Check sheet for the drawn part. Datum: minimum x, y, z corner. Units: mm. Coordinates: 2 decimals unless noted, no trailing zeros. Write each loop counter-clockwise with the first axis right and the second up, starting at its lowest first coordinate (ties: lowest second). Pieces come first, ordered by that corner, then holes. Notation, with made-up numbers: (6, 62) - (21, 62) arc R5 cw to (21, 71) - close; hole circle Ø7 at (-11, -0.5). An arc over 180 degrees is marked (long way). Write each question's results on one line, items separated by ' | '.
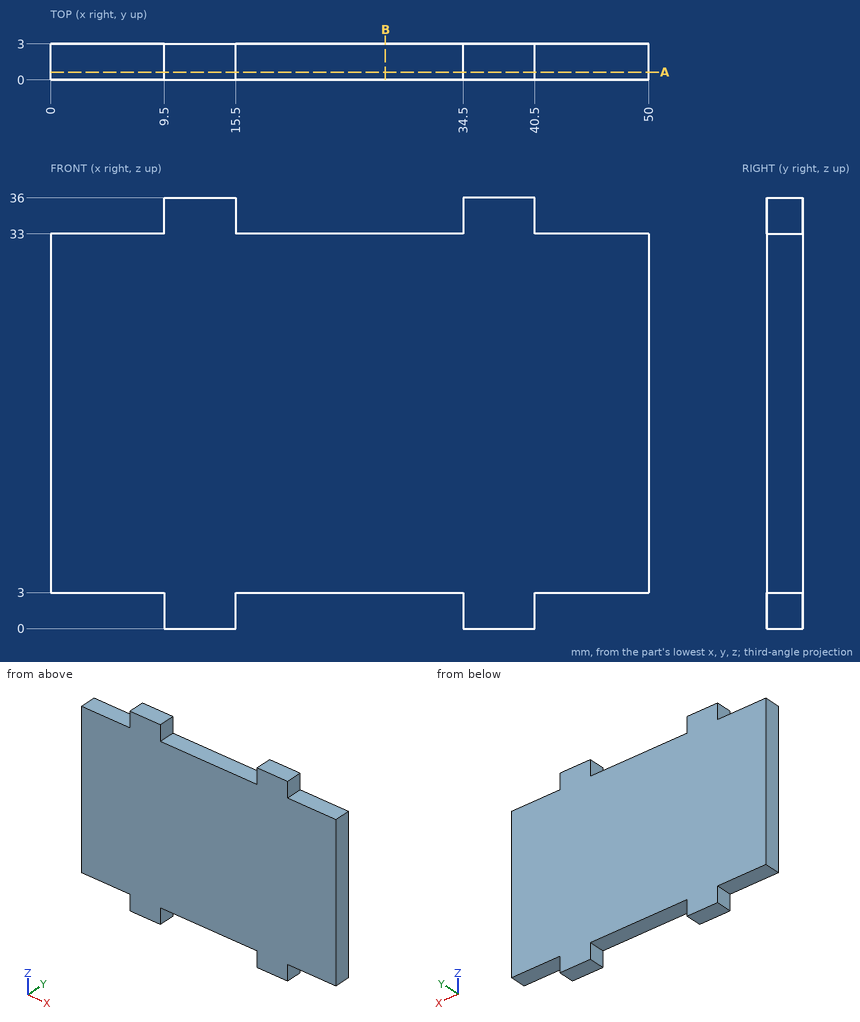
1. Go/stop test with flat-tipped pins: pin 1 (0.9 mm diameter, centred on y = 1, z = 34, fed in from +X); pin 2 (0.9 mm diameter, centred on x = 5, y = 1, fed in from -Z); pin 3 (1.5 mm diameter, centred on y = 2, z = 34.5, fed in from -X). Record where each tip stops, or that it passes through.
Values follow:
pin 1: stops at x = 40.5 | pin 2: stops at z = 3 | pin 3: stops at x = 9.5
2. Material ranges on L1, parallel to Z at x = 31, y = 1.3, recorded low to high. Write a range as [from, to].
Values follow:
L1: z = [3, 33]
3. Sectioned sample at B-B (x = 28). Record the cut outline in (y, z), then the cut area to 3 significant figures.
Values follow:
outline: (0, 3) - (3, 3) - (3, 33) - (0, 33) - close | area: 90.0 mm^2
4. Sectioned sample at A-A (y = 0.65). Record the cut outline in (x, z), then the cut area to 3 significant figures.
Values follow:
outline: (0, 3) - (9.5, 3) - (9.5, 0) - (15.5, 0) - (15.5, 3) - (34.5, 3) - (34.5, 0) - (40.5, 0) - (40.5, 3) - (50, 3) - (50, 33) - (40.5, 33) - (40.5, 36) - (34.5, 36) - (34.5, 33) - (15.5, 33) - (15.5, 36) - (9.5, 36) - (9.5, 33) - (0, 33) - close | area: 1,570 mm^2
